Model file for the job. Use its own axes, mm. A direction names the side the tool comes from. Coordinates: 2 decimals unless noted, no trailing zeros. Order: outer loops, then holes, each group sorted by start corner. A loop starts at its lowest first (then second) coordinate and runs counter-clockwise, first axis right, second up.
from build123d import *

# Parameters (mm, degrees)
SKETCH_1_R          = 1.525
EXTRUDE_1_DEPTH     = 5
CUT_EXTRUDE_START   = 3.5
CUT_EXTRUDE_1_DEPTH = 179.563175848
SKETCH_3_R          = 3
CUT_EXTRUDE_2_DEPTH = 2
EXTRUDE_2_DEPTH     = 5.95
SKETCH_7_R          = 1.525
CUT_EXTRUDE_3_DEPTH = 183.091741987
FILLET_4_R          = 4.5
CUT_EXTRUDE_4_DEPTH = 183.091741987
FILLET_5_R          = 2
FILLET_6_R          = 1


with BuildPart() as part:
    # 草图1 → 凸台-拉伸1 (new body)
    with BuildSketch(Plane(origin=(0, 0, 0), x_dir=(1, 0, 0), z_dir=(0, 1, 0))):
        with BuildLine():
            Line((21, 0), (21, -9.5))
            Line((21, -9.5), (54.333333333, -9.5))
            Line((54.333333333, -9.5), (61, -19))
            Line((61, -19), (65, -19))
            Line((65, -19), (175, -19))
            Line((175, -19), (181, -14))
            Line((181, -14), (181, -9.5))
            Line((181, -9.5), (75.433012702, -9.5))
            ThreePointArc((75.433012702, -9.5), (74.5, -9.25), (75.433012702, -9))
            Line((75.433012702, -9), (88, -9))
            Line((88, -9), (88, 0))
            Line((88, 0), (41.55, 0))
            Line((41.55, 0), (41.55, 9.5))
            Line((41.55, 9.5), (35, 9.5))
            Line((35, 9.5), (35, 0))
            Line((35, 0), (21, 0))
        make_face()
        with Locations(Location((25.75, -4.75, 0), (0, 0, 270))):
            Circle(SKETCH_1_R, mode=Mode.SUBTRACT)
    extrude(amount=EXTRUDE_1_DEPTH)

    # 草图2 → 切除-拉伸1 (cut, through all)
    with BuildSketch(Plane(origin=(0, 0, 0), x_dir=(1, 0, 0), z_dir=(0, 1, 0)).offset(CUT_EXTRUDE_START)):
        Polygon((75, -9), (75, 0), (88, 0), (88, -9), (75.433012702, -9), align=None)
        Polygon((75.433012702, -9.5), (175, -9.5), (173, -14), (77, -14), (75, -9.5), align=None)
    extrude(amount=CUT_EXTRUDE_1_DEPTH, mode=Mode.SUBTRACT)

    # 草图3 → 切除-拉伸2 (cut)
    with BuildSketch(Plane(origin=(0, 0, 0), x_dir=(1, 0, 0), z_dir=(0, 1, 0))):
        with Locations(Location((25.75, -4.75, 0), (0, 0, 270))):
            Circle(SKETCH_3_R)
    extrude(amount=CUT_EXTRUDE_2_DEPTH, mode=Mode.SUBTRACT)

    # 草图6 → 凸台-拉伸2 (add)
    with BuildSketch(Plane(origin=(0, 0, 0), x_dir=(1, 0, 0), z_dir=(0, 1, 0))):
        Polygon((173, -14), (173, -19), (175, -19), (181, -14), (181, -9.5), (175, -9.5), align=None)
    extrude(amount=EXTRUDE_2_DEPTH)

    # 草图7 → 切除-拉伸3 (cut, through all)
    with BuildSketch(Plane.XY):
        with Locations(Location((178, 2.975, 0), (0, 0, 180))):
            Circle(SKETCH_7_R)
    extrude(amount=CUT_EXTRUDE_3_DEPTH, mode=Mode.SUBTRACT)

    # 圆角4
    fillet_4_edges = [part.edges().sort_by_distance(p)[0] for p in [
        (21, 2.5, 9.5),
        (21, 2.5, 0),
    ]]
    fillet(fillet_4_edges, radius=FILLET_4_R)

    # 草图8 → 切除-拉伸4 (cut, through all)
    with BuildSketch(Plane(origin=(0, 0, 0), x_dir=(0, 0, -1), z_dir=(1, 0, 0))):
        Polygon((2.5, 5), (9.5, 2.5), (9.5, 5), align=None)
    extrude(amount=CUT_EXTRUDE_4_DEPTH, mode=Mode.SUBTRACT)

    # 圆角5
    fillet_5_edges = [part.edges().sort_by_distance(p)[0] for p in [
        (61, 2.5, 19),
        (54.333333333, 2.5, 9.5),
        (41.55, 2.5, 0),
    ]]
    fillet(fillet_5_edges, radius=FILLET_5_R)

    # 圆角6
    fillet_6_edges = [part.edges().sort_by_distance(p)[0] for p in [
        (35, 1.25, -9.5),
        (41.55, 1.25, -9.5),
        (38.275, 2.5, -9.5),
    ]]
    fillet(fillet_6_edges, radius=FILLET_6_R)


solid = part.part
Q1. Drop flat-ended pins along their axis: P1, Ø2.5, axis at x = 178, y = 2.975, coming from the -Z side; P2, Ø5, axis at x = 25.75, z = 4.75, coming from the -Y side; P3, Ø2.5, axis at x = 33, y = 2.5, coming from the +Z side; P4, Ø6, axis at x = 63.5, z = 8, coming from the +Y side. Give the stop position or say it passes through.
Established:
P1: passes through
P2: stops at y = 2
P3: stops at z = 9.5
P4: stops at y = 5
Q2. Which spindle directions (+Z, -Z, +X, -X, +Y, -Y) get a long thin tool onto all of the face, cutting with end or side? Do faces 5 (the face through (82, 2, 9)), 6 (the face through (66, 2, 0)), 7 (the face through (30, 2, 0)). Say none if no direction does.
Established:
face 5: +X, +Y, -Y
face 6: -Z, +X, +Y, -Y
face 7: -Z, -X, +Y, -Y
Q3. Cut at A-A, the plane x = 178. List the corners of the cut face in (y, z), plus the area to 3 significant figures.
Established:
outline: (0, 9.5) - (1.45, 9.5) - (1.45, 16.5) - (0, 16.5) - close; (4.5, 9.5) - (5.95, 9.5) - (5.95, 16.5) - (4.5, 16.5) - close
area: 20.3 mm2
Q4. Cut at C-C, the plane z = 15.5. List the corners of the cut face in (x, y) (3 decimals).
Established:
outline: (58.544, 0) - (179.2, 0) - (179.2, 2.034) arc R1.525 cw (long way) to (179.2, 3.916) - (179.2, 5.95) - (173, 5.95) - (173, 5) - (58.544, 5) - close
Q5. Cut at D-D, the plane x = 39. List the corners of the cut face in (y, z), plus the area to 3 significant figures.
Established:
outline: (0, -9.5) - (1.8, -9.5) arc R1 ccw to (2.74, -8.84) - (5, -2.5) - (5, 9.5) - (0, 9.5) - close
area: 86.2 mm2
Q6. Mould opens along Y. For faces 1 (the face through (100, 0, 11)), 2 (the face through (22.353, 2.535, 1.283)), 3 (the face through (176.545, 2.517, 12.659)), 4 (the face through (126, 3.5, 12)) say: pulls with the +Y half, pulls with the -Y half, needs draft (parallel to the pull), parting line crosses it, or undercut.
Established:
face 1: pulls with the -Y half
face 2: needs draft
face 3: undercut
face 4: pulls with the +Y half
Q7. Probe line 1 (Z direction, x = 25.75, y = 3.55) (3 decimals); line 2 (X direction, y = 2.9, z = 4.75) (3 decimals); line 3 (Y direction, x = 178, z = 13.5). List the from-to ranges inside material, lowest first.
Established:
line 1: z = 0 to 3.225, 6.275 to 9.5
line 2: x = 21 to 24.225, 27.275 to 88
line 3: y = 0 to 1.45, 4.5 to 5.95
Q8. Cut at B-B, the plane x = 90. List the corners of the cut face in (y, z).
Established:
outline: (0, 9.5) - (3.5, 9.5) - (3.5, 14) - (5, 14) - (5, 19) - (0, 19) - close
